Part print with two shaded views. Sizes in mm from the minimum x, y, z corner. A direction names the side the tool comes from. Give positions to 0.01 mm unless a question says otherwise; leave off trailing zeros. Order: outer loops, then holes, each group sorted by start corner. A loop starts at its lowest first (then second) coordinate and runs counter-clockwise, first axis right, second up.
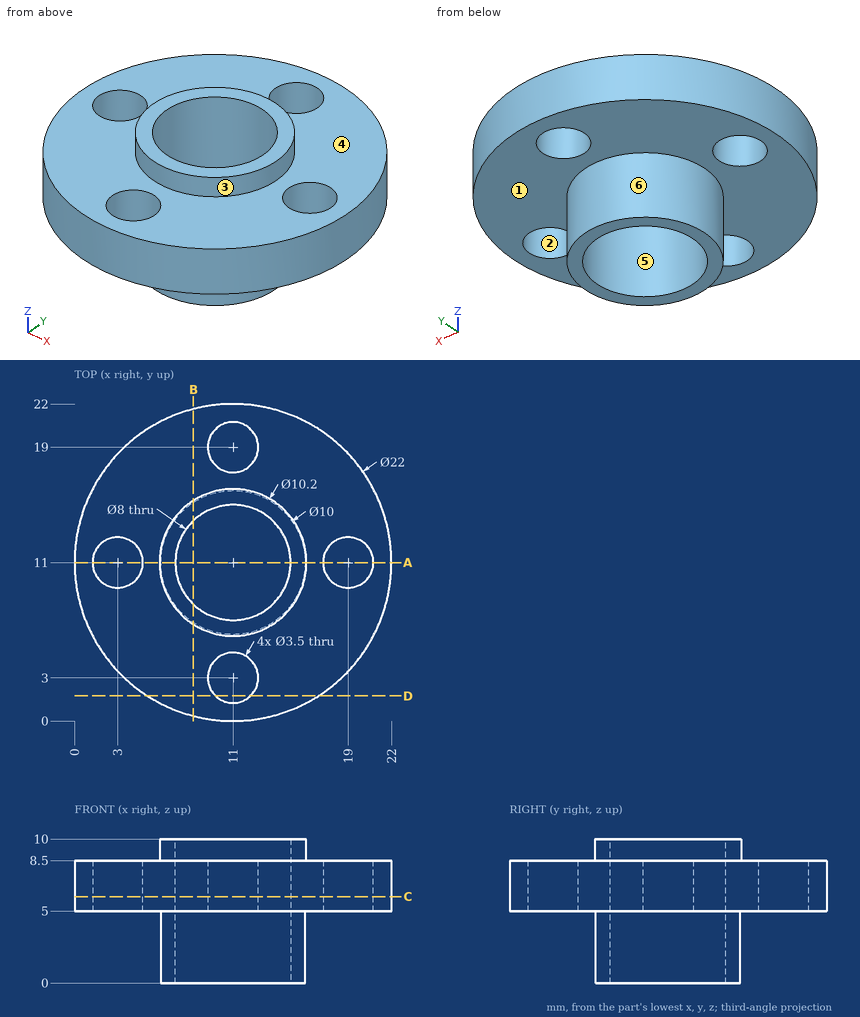
Item 1: Drop flat-ended pins along their axis: pin 1 Ø6 at (x, y) = (20, 10) entering from -Z; pin 2 Ø4.5 at (x, y) = (11, 19) entering from +Z; pin 3 Ø1 at (y, z) = (4.5, 5) entering from -X; pin 4 Ø2 at (x, y) = (11, 3) entering from +Z. Give the stop position or say it passes through.
Item 2: Slice it at A-A (y = 11). Give the cut face in (x, z), and give its area (3 significant figures).
Item 3: Slice it at B-B (x = 8.25). Give the cut face in (y, z).
Item 4: Wall check: L1, parallel to Z at x = 7, y = 5.25; L2, parallel to Y at x = 14.5, z = 4; L3, parallel to Y at x = 3, z = 7.6. Give the ranges that are in metal, low to high.
Item 5: Slice it at D-D (y = 1.75). Give the cut face in (x, z), and give its area (3 significant figures).
Item 6: Slice it at C-C (z = 6). Give the cut face in (x, y).
Item 7: Two-plate mould, pull along X, no slides. Class the marked faces 1, 2 and 3: released by +X, released by -X, zero draft, split by the parting line, or undercut.
Item 8: Tool access for the marked faces 4, 5 and 6: list every direction of +Z, -Z, +X, -X, +Y, -Y with a clear straight run to the whole face (end or side of a thin tool).
A:
1. pin 1: stops at z = 5
1. pin 2: stops at z = 8.5
1. pin 3: stops at x = 1.78
1. pin 4: passes through
2. outline: (0, 5) - (1.25, 5) - (1.25, 8.5) - (0, 8.5) - close; (4.75, 5) - (6, 5) - (6, 0) - (7, 0) - (7, 10) - (5.9, 10) - (5.9, 8.5) - (4.75, 8.5) - close; (15, 0) - (16, 0) - (16, 5) - (17.25, 5) - (17.25, 8.5) - (16.1, 8.5) - (16.1, 10) - (15, 10) - close; (20.75, 5) - (22, 5) - (22, 8.5) - (20.75, 8.5) - close
2. area: 37.8 mm2
3. outline: (0.35, 5) - (6.82, 5) - (6.82, 0) - (8.1, 0) - (8.1, 10) - (6.7, 10) - (6.7, 8.5) - (0.35, 8.5) - close; (13.9, 0) - (15.18, 0) - (15.18, 5) - (21.65, 5) - (21.65, 8.5) - (15.3, 8.5) - (15.3, 10) - (13.9, 10) - close
4. L1: z = 5 to 8.5
4. L2: y = 7.43 to 9.06, 12.94 to 14.57
4. L3: y = 3.45 to 9.25, 12.75 to 18.55
5. outline: (5.05, 5) - (9.78, 5) - (9.78, 8.5) - (5.05, 8.5) - close; (12.22, 5) - (16.95, 5) - (16.95, 8.5) - (12.22, 8.5) - close
5. area: 33.1 mm2
6. outline: circle Ø22 at (11, 11); hole circle Ø3.5 at (3, 11); hole circle Ø8 at (11, 11); hole circle Ø3.5 at (11, 3); hole circle Ø3.5 at (11, 19); hole circle Ø3.5 at (19, 11)
7. face 1: zero draft
7. face 2: undercut
7. face 3: split by the parting line
8. face 4: +Z
8. face 5: +Z, -Z
8. face 6: -Z
